Could you check a few things on this model? Use its own coordinates, in mm. A direction names the side the tool comes from. Coordinates: 2 decimals unless noted, no trailing zeros. Write each loop counter-clockwise with the first axis right and the second up, starting at its lowest first coordinate (ties: lowest second). Pieces come first, ordered by that corner, then holes.
Item 1: For P1, Ø1, axis at y = -5.5, z = -17, coming from the -X side; P2, Ø2, axis at y = 5, z = 6, coming from the +X side; P3, Ø10.5, axis at x = 0.5, y = -3, coming from the +Z side (3 decimals); P4, Ø10, axis at y = -8.5, z = -14, coming from the -X side, each with a flat end and sliding along its axis, tell me the tip position at first contact or that it passes through.
Item 2: Thinking about a two-plate mould opening in X: for faces 3 (the cylindrical face through (10.6, 3.34, 1.53)), 4 (the cylindrical face through (-3.78, -2.9, -1.25)), 5 (the flat face through (4.02, -7.1, -4.381)), which applies, +X half, -X half, draft (parallel to the pull), parting line (faces both ways), or undercut?
Item 3: I want a section at A-A on z = -9.5. Please give me the cut outline in (x, y) (1 decimal).
Item 4: If I drill on probe 1 along Y at (x, z) = (0, -3); probe 2 along Y at (x, z) = (2, -1.5); probe 3 along X at (y, z) = (-1.5, 20.5), over which ranges is the centre line in solid material (lowest first)?
Item 5: Which directions (+Z, -Z, +X, -X, +Y, -Y) give clear straight access to the entire face, cutting with the end or side of a thin tool? Please do faces 1 (the flat face through (0, -5, -25.4)), 2 (the cylindrical face through (1.73, -7.81, 11.2)).
from build123d import *

# Parameters (mm, degrees)
SKETCH1_R                  = 11.1125
SKETCH1_R_2                = 3.2004
EXTRUDE1_DEPTH             = 25.4
SKETCH5_R                  = 11.1125
SKETCH5_R_2                = 3.2004
CUT_EXTRUDE1_DEPTH         = 3.175
SKETCH6_R                  = 4.7625
CUT_EXTRUDE2_DEPTH         = 48.625
CUT_EXTRUDE3_START         = -1.5875
SKETCH7_R                  = 11.1125
SKETCH7_R_2                = 8.001
CUT_EXTRUDE3_DEPTH         = 5.334
CHAMFER2_SIZE              = 0.381
LPATTERN1_COUNT            = 6
LPATTERN1_PITCH            = 6.477
CHAMFER2_OF_LPATTERN1_SIZE = 0.381


with BuildPart() as part:
    # Sketch1 → Extrude1 (new body, symmetric)
    with BuildSketch(Plane.XY):
        Circle(SKETCH1_R)
        Circle(SKETCH1_R_2, mode=Mode.SUBTRACT)
    extrude(amount=EXTRUDE1_DEPTH, both=True)

    # Sketch5 → Cut-Extrude1 (cut)
    with BuildSketch(Plane.XY.offset(25.4)):
        Circle(SKETCH5_R)
        Circle(SKETCH5_R_2, mode=Mode.SUBTRACT)
    extrude(amount=-CUT_EXTRUDE1_DEPTH, mode=Mode.SUBTRACT)

    # Sketch6 → Cut-Extrude2 (cut, through all)
    with BuildSketch(Plane.XY.offset(22.225)):
        Circle(SKETCH6_R)
    extrude(amount=-CUT_EXTRUDE2_DEPTH, mode=Mode.SUBTRACT)

    # Sketch7 → Cut-Extrude3 (cut)
    with BuildSketch(Plane(origin=(0, 0, -25.4), x_dir=(-1, 0, 0), z_dir=(0, 0, -1)).offset(CUT_EXTRUDE3_START)):
        Circle(SKETCH7_R)
        Circle(SKETCH7_R_2, mode=Mode.SUBTRACT)
    cut_extrude3 = extrude(amount=-CUT_EXTRUDE3_DEPTH, mode=Mode.SUBTRACT)

    # Chamfer2
    chamfer2_edges = [part.edges().sort_by_distance(p)[0] for p in [
        (-11.1125, 0, -18.4785),
        (-11.1125, 0, -23.8125),
    ]]
    chamfer(chamfer2_edges, length=CHAMFER2_SIZE)

    # LPattern1: Cut-Extrude3 ×6
    with Locations(*[(0, 0, i * LPATTERN1_PITCH) for i in range(1, LPATTERN1_COUNT)]):
        add(cut_extrude3, mode=Mode.SUBTRACT)

    # Chamfer2 of LPattern1
    chamfer2_of_lpattern1_edges = [part.edges().sort_by_distance(p)[0] for p in [
        (-11.1125, 0, -12.0015),
        (-11.1125, 0, -17.3355),
        (-11.1125, 0, -5.5245),
        (-11.1125, 0, -10.8585),
        (-11.1125, 0, 0.9525),
        (-11.1125, 0, -4.3815),
        (-11.1125, 0, 7.4295),
        (-11.1125, 0, 2.0955),
        (-11.1125, 0, 13.9065),
        (-11.1125, 0, 8.5725),
    ]]
    chamfer(chamfer2_of_lpattern1_edges, length=CHAMFER2_OF_LPATTERN1_SIZE)


solid = part.part
Response values:
1. P1: stops at x = -9.47
1. P2: stops at x = 6.93
1. P3: stops at z = 22.225
1. P4: stops at x = -10.33
2. face 3: parting line
2. face 4: undercut
2. face 5: draft
3. outline: circle Ø16 at (0, 0); hole circle Ø9.5 at (0, 0)
4. probe 1: y = -8 to -4.76, 4.76 to 8
4. probe 2: y = -7.75 to -4.32, 4.32 to 7.75
4. probe 3: x = -11.01 to -4.52, 4.52 to 11.01
5. face 1: -Z, +X, -X, +Y, -Y
5. face 2: none
